Here's how the part is built. I have some questions about the finished solid (model axes, mm). A direction names the side the tool comes from. Round coordinates to 2 decimals unless told otherwise and drop trailing zeros. Order: outer loops, then holes, each group sorted by start corner. A loop starts at its lowest first (then second) coordinate and runs counter-clockwise, first axis right, second up. Notation, with made-up numbers: M 82,-19.75 L 87,-19.75 A35 cw 87,17.25 Z; hole C 68,-11.75 d4. An arc over 180 degrees is marked long. Write each question's results on one line, items separated by ' | '. Start each with the question number.
Autodesk Inventor part; units mm, degrees
ref_plane "Work Plane1" through (0, -150, 0) normal (0, -1, 0) x (1, 0, 0)
ref_plane "Work Plane3" through (-644.8193, 10, 570.5647) normal (0, 0, 1) x (1, 0, 0)
ref_plane "Work Plane4" through (-644.8193, 10, 295.5647) normal (0, 0, 1) x (1, 0, 0)
sketch "Sketch1" plane through (0, 0, 0) normal (0, 1, 0) x (-1, 0, 0)
  line L0 (65.8193, -27.9353) -> (65.8193, 275.5647)
  line L1 (65.8193, 275.5647) -> (634.8193, 275.5647)
  line L2 (634.8193, 275.5647) -> (634.8193, -27.9353)
  line L3 (448.3193, 71.0647) -> (252.3193, 71.0647)
  line L4 (448.3193, 71.0647) -> (448.3193, -27.9353)
  line L5 (252.3193, 71.0647) -> (252.3193, -27.9353)
  line L6 (65.8193, -27.9353) -> (252.3193, -27.9353)
  line L7 (448.3193, -27.9353) -> (634.8193, -27.9353)
  point P0 (0, 0)
  dimension "d0" = 569
  dimension "d1" = 303.5
  dimension "d2" = 196
  dimension "d3" = 186.5
  dimension "d4" = 99
extrude "Extrusion1" add sketch "Sketch1" along normal blind 10
sketch "Sketch2" plane through (0, 0, 0) normal (0, -1, 0) x (1, 0, 0)
  line L0 (-65.8193, 275.5647) -> (-65.8193, -27.9353)
  line L1 (-65.8193, 275.5647) -> (-65.8193, -27.9353)
  line L2 (-65.8193, -27.9353) -> (-55.8193, -27.9353)
  line L3 (-55.8193, -27.9353) -> (-55.8193, 275.5647)
  line L4 (-55.8193, 275.5647) -> (-65.8193, 275.5647)
  line L5 (-634.8193, 275.5647) -> (-65.8193, 275.5647)
  line L6 (-634.8193, -27.9353) -> (-634.8193, 275.5647)
  line L7 (-634.8193, 275.5647) -> (-634.8193, -27.9353)
  line L8 (-634.8193, -27.9353) -> (-644.8193, -27.9353)
  line L9 (-644.8193, -27.9353) -> (-644.8193, 275.5647)
  line L10 (-644.8193, 275.5647) -> (-634.8193, 275.5647)
  point P0 (0, 0)
  dimension "d7" = 10
  dimension "d8" = 10
extrude "Extrusion2" add sketch "Sketch2" along normal blind 300
extrude "Extrusion3" add sketch "Sketch2" against normal blind 10
sketch "Sketch3" plane through (0, 0, 0) normal (0, -1, 0) x (1, 0, 0)
  line L0 (-252.3193, -27.9353) -> (-65.8193, -27.9353)
  line L1 (-252.3193, -27.9353) -> (-65.8193, -27.9353)
  line L2 (-65.8193, -27.9353) -> (-65.8193, -37.9353)
  line L3 (-65.8193, -37.9353) -> (-252.3193, -37.9353)
  line L4 (-252.3193, -37.9353) -> (-252.3193, -27.9353)
  line L5 (-448.3193, 71.0647) -> (-448.3193, -27.9353)
  line L6 (-448.3193, -37.9353) -> (-448.3193, -27.9353)
  line L7 (-634.8193, -27.9353) -> (-634.8193, 275.5647)
  line L8 (-448.3193, -27.9353) -> (-634.8193, -27.9353)
  line L9 (-634.8193, -27.9353) -> (-634.8193, -37.9353)
  line L10 (-634.8193, -37.9353) -> (-448.3193, -37.9353)
  point P0 (0, 0)
  point P1 (-644.8193, -27.9353)
  point P2 (-541.5693, -37.9353)
  point P3 (-159.0693, -37.9353)
  point P4 (-448.3193, -32.9353)
  dimension "d13" = 10
extrude "Extrusion4" add sketch "Sketch3" against normal blind 10
extrude "Extrusion5" add sketch "Sketch3" along normal blind 300
ref_plane "Work Plane1" through (0, -150, 0) normal (0, -1, 0) x (1, 0, 0)
mirror "Mirror1" about plane through (0, -150, 0) normal (0, -1, 0) of "Extrusion1", "Extrusion4", "Extrusion3"
sketch "Sketch4" plane through (-644.8193, 10, -27.9353) normal (-1, 0, 0) x (0, 0, 1)
  circle A0 centre (95, -172.6482) radius 20
  line L0 (0, 0) -> (0, -320)
  point P0 (27.9353, -10)
  dimension "d20" = 40
  dimension "d21" = 95
extrude "Extrusion6" cut sketch "Sketch4" against normal through all
sketch "Sketch5" plane through (0, 10, 0) normal (0, 1, 0) x (1, 0, 0)
  line L0 (-65.8193, -275.5647) -> (-634.8193, -275.5647)
  line L1 (-644.8193, 27.9353) -> (-644.8193, -275.5647)
  line L2 (-644.8193, -220.5647) -> (-519.8193, -220.5647)
  line L3 (-644.8193, -275.5647) -> (-55.8193, -275.5647)
  line L4 (-55.8193, -275.5647) -> (-55.8193, 27.9353)
  line L5 (-55.8193, -220.5647) -> (-55.8193, -275.5647)
  line L6 (-464.8193, -275.5647) -> (-55.8193, -275.5647)
  line L7 (-464.8193, -275.5647) -> (-644.8193, -275.5647)
  line L8 (-644.8193, -275.5647) -> (-644.8193, -220.5647)
  line L9 (-55.8193, -220.5647) -> (-519.8193, -220.5647)
  point P0 (0, 0)
  point P1 (-118.3193, -220.5647)
  point P2 (-582.3193, -220.5647)
  dimension "d27" = 125
extrude "Extrusion7" cut sketch "Sketch5" against normal through all
ref_plane "Work Plane3" through (-644.8193, 10, 570.5647) normal (0, 0, 1) x (1, 0, 0)
ref_plane "Work Plane4" through (-644.8193, 10, 295.5647) normal (0, 0, 1) x (1, 0, 0)
sketch "Sketch9" plane through (-644.8193, 10, 295.5647) normal (0, 0, 1) x (1, 0, 0)
  line L0 (146.5, -320) -> (146.5, 0)
  line L1 (146.5, 0) -> (442.5, 0)
  line L2 (442.5, 0) -> (442.5, -320)
  line L3 (442.5, -320) -> (146.5, -320)
  line L4 (10, -310) -> (579, -310) construction
  line L5 (392.5, -10) -> (392.5, -310) construction
  line L6 (579, -10) -> (10, -10) construction
  line L7 (0, 0) -> (589, 0) construction
  line L8 (156.5, -10) -> (156.5, -310) construction
  line L9 (156.5, -310) -> (432.5, -310) construction
  line L10 (432.5, -310) -> (432.5, -10) construction
  line L11 (432.5, -10) -> (156.5, -10) construction
  point P0 (644.8193, -10)
  point P1 (146.5, -160)
  point P2 (392.5, -160)
  point P3 (294.5, -10)
  point P4 (294.5, 0)
  point P5 (294.5, 0)
  point P6 (294.5, -320)
  dimension "d50" = 296
  dimension "d51" = 10
sketch "Sketch10" plane through (-644.8193, 10, 570.5647) normal (0, 0, 1) x (1, 0, 0)
  line L0 (269.5, -185) -> (319.5, -185)
  line L1 (319.5, -185) -> (319.5, -135)
  line L2 (319.5, -135) -> (269.5, -135)
  line L3 (269.5, -135) -> (269.5, -185)
  line L4 (196.5, -10) -> (196.5, -310)
  line L5 (579, -10) -> (10, -10)
  line L6 (279.5, -175) -> (279.5, -145) construction
  line L7 (279.5, -145) -> (309.5, -145) construction
  line L8 (309.5, -145) -> (309.5, -175) construction
  line L9 (309.5, -175) -> (279.5, -175) construction
  point P0 (644.8193, -10)
  point P1 (269.5, -160)
  point P2 (196.5, -160)
  point P3 (294.5, -135)
  point P4 (294.5, -10)
  dimension "d52" = 50
  dimension "d53" = 50
  dimension "d54" = 10
loft "Loft3" add profiles "Sketch9" section 1 edges at (-350.3193, -310, 220.5647) (-55.8193, -150, 220.5647) (-350.3193, 10, 220.5647) (-644.8193, -150, 220.5647)
sketch "Sketch11" plane through (-644.8193, 10, 295.5647) normal (0, 0, 1) x (1, 0, 0)
  line L0 (146.5, -320) -> (442.5, -320) construction
  line L1 (442.5, -320) -> (442.5, 0) construction
  line L2 (442.5, 0) -> (146.5, 0) construction
  line L3 (146.5, 0) -> (146.5, -320) construction
  line L4 (432.5, -10) -> (432.5, -310)
  line L5 (432.5, -310) -> (156.5, -310)
  line L6 (156.5, -310) -> (156.5, -10)
  line L7 (156.5, -10) -> (432.5, -10)
  point P0 (644.8193, -10)
  dimension "d59" = 10
loft "Loft4" cut profiles "Sketch11" section 1 edges at (-350.3193, -300, 220.5647) (-634.8193, -150, 220.5647) (-350.3193, 0, 220.5647) (-65.8193, -150, 220.5647)
loft "Loft5" add profiles "Sketch10" section 1 edges at (-350.3193, -310, 295.5647) (-202.3193, -150, 295.5647) (-350.3193, 10, 295.5647) (-498.3193, -150, 295.5647)
sketch "Sketch12" plane through (-644.8193, 10, 570.5647) normal (0, 0, 1) x (1, 0, 0)
  line L0 (309.5, -175) -> (309.5, -145)
  line L1 (309.5, -145) -> (279.5, -145)
  line L2 (279.5, -145) -> (279.5, -175)
  line L3 (279.5, -175) -> (309.5, -175)
  line L4 (319.5, -185) -> (269.5, -185)
  line L5 (319.5, -135) -> (319.5, -185)
  point P0 (644.8193, -10)
  point P1 (294.5, -175)
  point P2 (294.5, -185)
  point P3 (309.5, -160)
  point P4 (319.5, -160)
  dimension "d69" = 30
  dimension "d70" = 30
loft "Loft6" cut profiles "Sketch12" section 1 edges at (-212.3193, -150, 295.5647) (-350.3193, -300, 295.5647) (-488.3193, -150, 295.5647) (-350.3193, 0, 295.5647)
extrude "Extrusion9" add sketch "Sketch10" against normal blind 10 draft 10
properties part number "armorMk1"
(1) I want a section at B-B on x = -609. Write out the boundary of the cut face in (y, z), and give its area (3 significant figures).
(2) On a 3-axis mill with a long thin cutter (end or side, diameter ignored), from which of +Z, -Z, +X, -X, +Y, -Y can I reach the whole of each face in a straight line? I mean faces 4 (the flat face through (-448.319, -149.3, -28.1)), 5 (the flat face through (-160, -148, -27.935)), 6 (the flat face through (-351, -150, 560.565)). Say none if no direction works.
(3) Please list where these lines run through material, in increasing order: line 1 (X direction, y = -53, z = 63.5); line 2 (Y direction, x = -366, z = 192); line 3 (Z direction, x = -473, y = -108.5).
(4) If we mould it in two halves opening along Y, with no side actions, what happens to faces 1 (the flat face through (-346, 0, 136)), 2 (the flat face through (-346, -310, 131)), 3 (the flat face through (-160, -148, -37.935))? For each: pulls with the +Y half, pulls with the -Y half, needs draft (parallel to the pull), parting line crosses it, or undercut.
(5) I want a section at C-C on z = 257. Write out the boundary of the cut face in (x, y), and give its area (3 significant figures).
(6) I'm going to push flat-ended pins straight in: pin 1 Ø11 at (y, z) = (-222.5, -35) entering from -X; pin 2 Ø5 at (x, y) = (-307.5, -303.5) entering from -Z; pin 3 Ø11 at (y, z) = (-220, -35) entering from +X. Where does each tip first touch, or does it pass through?
(7) I want a section at A-A on z = -1. Write out the boundary of the cut face in (x, y), and give its area (3 significant figures).
Solutions:
1) outline: M -310,-37.94 L 10,-37.94 L 10,238.9 L -310,238.9 Z; hole M -300,-27.94 L 0,-27.94 L 0,233.78 L -300,233.78 Z | area: 10,100 mm^2
2) face 4: -Z, +Y, -Y | face 5: none | face 6: -Z
3) line 1: -644.82 to -634.82, -65.82 to -55.82 | line 2: -310 to -300, 0 to 10 | line 3: -37.94 to -27.94, 329.82 to 352.17
4) face 1: undercut | face 2: pulls with the -Y half | face 3: needs draft
5) outline: M -573.65,-310 L -126.99,-310 L -126.99,10 L -573.65,10 Z; hole M -563.65,-300 L -136.99,-300 L -136.99,0 L -563.65,0 Z | area: 14,900 mm^2
6) pin 1: x = -634.82 | pin 2: z = 71.06 | pin 3: x = -65.82
7) outline: M -644.82,-310 L -448.32,-310 L -448.32,-300 L -634.82,-300 L -634.82,0 L -448.32,0 L -448.32,10 L -644.82,10 Z; M -252.32,-310 L -55.82,-310 L -55.82,10 L -252.32,10 L -252.32,0 L -65.82,0 L -65.82,-300 L -252.32,-300 Z | area: 13,900 mm^2
